Geometry check sheet. Reference: the model listing, model coordinates, mm. Give positions to 0.01 mm unless a question says otherwise; leave off trailing zeros. Write each loop counter-clockwise with the first axis right and the second up, starting at its lowest first coordinate (ties: lowest second). Pieces come first, ordered by that corner, then holes. Notation, with made-up numbers: (89.25, -21.5) - (107.25, -21.5) arc R8 ccw to (107.25, -9.5) - close; hole circle Ø10 at (23, 31). An arc over 180 degrees is marked (long way). Use a Markdown table: item, result.
```python
from build123d import *

# Parameters (mm, degrees)
SKETCH_1_W          = 11.9
SKETCH_1_H          = 11.9
SKETCH_1_R          = 5.05
EXTRUDE_1_DEPTH     = 2.8
CHAMFER_1_SIZE      = 0.9
SKETCH1_OUTSIDE_W   = 17.312
SKETCH1_OUTSIDE_H   = 17.312
SKETCH1_OUTSIDE_W_2 = 11.3
SKETCH1_OUTSIDE_H_2 = 11.4
CUT_EXTRUDE1_DEPTH  = 9.868201622
SKETCH2_R           = 5.15
CUT_EXTRUDE2_DEPTH  = 9.500147058


with BuildPart() as part:
    # 草图1 → 凸台-拉伸1 (new body)
    with BuildSketch(Plane(origin=(0, 0, 0), x_dir=(1, 0, 0), z_dir=(0, 1, 0))):
        Rectangle(SKETCH_1_W, SKETCH_1_H)
        with Locations(Location((0, 0, 0), (0, 0, 270))):
            Circle(SKETCH_1_R, mode=Mode.SUBTRACT)
    extrude(amount=EXTRUDE_1_DEPTH)

    # 倒角1
    chamfer_1_edges = [part.edges().sort_by_distance(p)[0] for p in [
        (0, 2.8, -5.05),
    ]]
    chamfer(chamfer_1_edges, length=CHAMFER_1_SIZE - 0.0001)  # a hair under: the kernel refuses the full size

    # Sketch1 outside → Cut-Extrude1 (cut, through all)
    with BuildSketch(Plane(origin=(0, 2.8, 0), x_dir=(1, 0, 0), z_dir=(0, 1, 0))):
        Rectangle(SKETCH1_OUTSIDE_W, SKETCH1_OUTSIDE_H)
        Rectangle(SKETCH1_OUTSIDE_W_2, SKETCH1_OUTSIDE_H_2, mode=Mode.SUBTRACT)
    extrude(amount=-CUT_EXTRUDE1_DEPTH, mode=Mode.SUBTRACT)

    # Sketch2 → Cut-Extrude2 (cut, through all)
    with BuildSketch(Plane(origin=(0, 2.8, 0), x_dir=(1, 0, 0), z_dir=(0, 1, 0))):
        with Locations(Location((0, 0, 0), (0, 0, 270))):
            Circle(SKETCH2_R)
    extrude(amount=-CUT_EXTRUDE2_DEPTH, mode=Mode.SUBTRACT)


solid = part.part
```
1) Mould release check, pull along X, two halves, no side actions. Record for faces 1 (the flat face through (-5, 2.8, 4)), 2 (the flat face through (5.65, 1, 0)), 3 (the conical face through (-2.026, 2.139, 4.886)), 4 (the cylindrical face through (-5.028, 1.014, -1.116)): pulls with the +X half, pulls with the -X half, needs draft (parallel to the pull), parting line crosses it, or undercut.
Working result:
| item | result |
|---|---|
| face 1 | needs draft |
| face 2 | pulls with the +X half |
| face 3 | undercut |
| face 4 | undercut |
2) Section check B-B on x = 0. Record the boundary of the cut face in (y, z), then the cut area to 3 significant figures.
Working result:
| item | result |
|---|---|
| outline | (0, -5.7) - (2.55, -5.7) - (2, -5.15) - (0, -5.15) - close; (0, 5.15) - (2, 5.15) - (2.55, 5.7) - (0, 5.7) - close |
| area | 2.50 mm² |
3) Section check C-C on z = 0. Record the boundary of the cut face in (x, y), then the cut area to 3 significant figures.
Working result:
| item | result |
|---|---|
| outline | (-5.65, 0) - (-5.15, 0) - (-5.15, 2) - (-5.65, 2.5) - close; (5.15, 0) - (5.65, 0) - (5.65, 2.5) - (5.15, 2) - close |
| area | 2.25 mm² |
4) Section check A-A on y = 1.85. Record the boundary of the cut face in (x, z), then the cut area to 3 significant figures.
Working result:
| item | result |
|---|---|
| outline | (-5.65, -5.7) - (5.65, -5.7) - (5.65, 5.7) - (-5.65, 5.7) - close; hole circle Ø10.3 at (0, 0) |
| area | 45.5 mm² |
5) Depth check by flat-ended pin: P1, Ø6, axis at x = -0.5, z = 1.5, coming from the -Y side. Enter the tip coordinate at first touch or a pass-through.
Working result:
| item | result |
|---|---|
| P1 | passes through |
6) Material ranges on L1, parallel to X at y = 0.75, z = 0; L2, parallel to Z at x = -0.75, y = 2.3; L3, parallel to Z at x = -3.75, y = 1.95, recorded low to high. Write a range as from..to.
Working result:
| item | result |
|---|---|
| L1 | x = -5.65..-5.15, 5.15..5.65 |
| L2 | z = -5.7..-5.4, 5.4..5.7 |
| L3 | z = -5.7..-3.53, 3.53..5.7 |
